Answer from the drawing. Dimensions are ordinates in mm from the lowest x, y and z of the part. A direction names the side the tool comes from. Give positions to 0.01 mm unless a question says otherwise; leave off trailing zeros. Order: outer loops, then holes, each group sorted by start corner. A loop starts at its lowest first (then second) coordinate and runs counter-clockwise, first axis right, second up. Notation, with made-up numbers: (64, 16) - (106, 16) arc R24 cw to (106, 32) - close; hole circle Ø9 at (74, 54.5). An arc over 180 degrees is marked (long way). Answer in a Markdown table with one row per item.
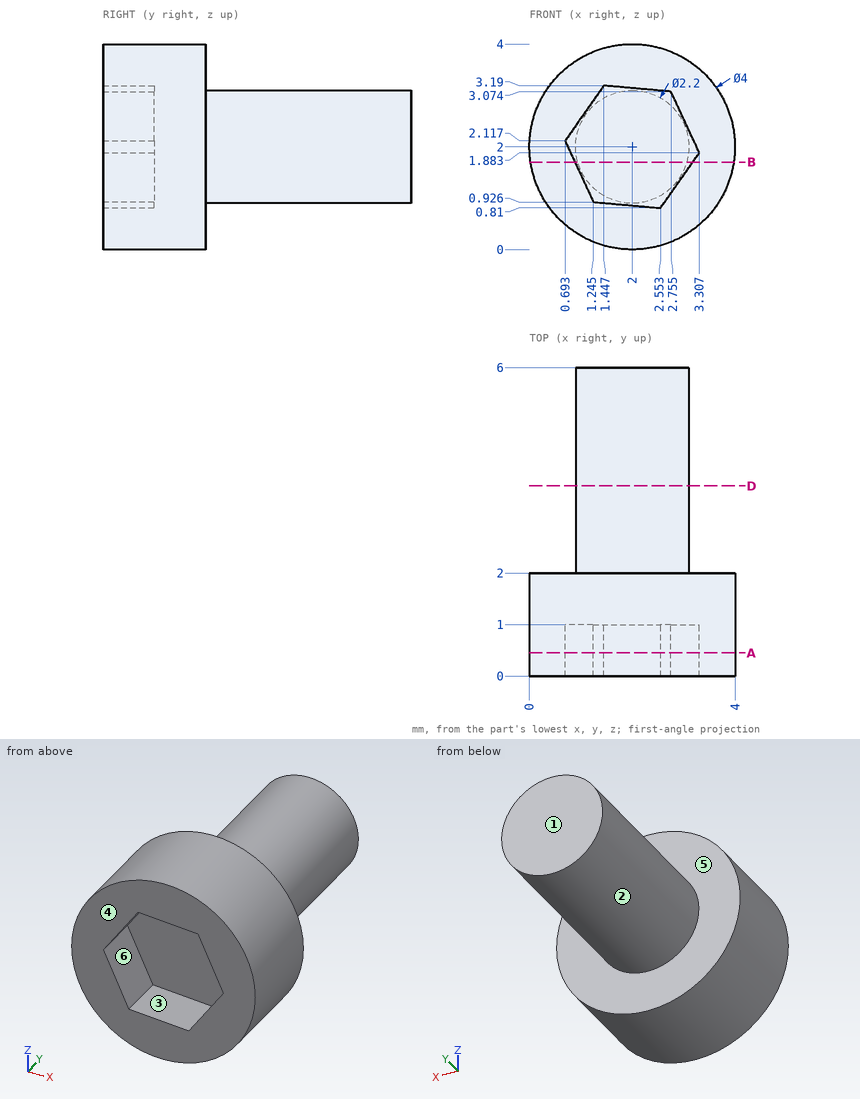
Item 1: Consider line 1 (Y direction, x = 1.2, z = 1.35); line 2 (Y direction, x = 3.4, z = 2.3); line 3 (Z direction, x = 1.2, y = 3.4) (1 decimal). Determine where each line is inside the solid, lowest interval first.
Answer block:
| item | result |
|---|---|
| line 1 | 1 to 6 |
| line 2 | 0 to 2 |
| line 3 | 1.2 to 2.8 |
Item 2: Find section B-B on z = 1.7. Write down the section's boundary in (x, y).
Answer block:
| item | result |
|---|---|
| outline | (0.02, 0) - (0.89, 0) - (0.89, 1) - (3.18, 1) - (3.18, 0) - (3.98, 0) - (3.98, 2) - (3.06, 2) - (3.06, 6) - (0.94, 6) - (0.94, 2) - (0.02, 2) - close |
Item 3: Find section A-A on y = 0.45. Write down the section's boundary in (x, z) (1 decimal).
Answer block:
| item | result |
|---|---|
| outline | circle Ø4 at (2, 2); hole (0.7, 2.1) - (1.2, 0.9) - (2.6, 0.8) - (3.3, 1.9) - (2.8, 3.1) - (1.4, 3.2) - close |
Item 4: Each of these flat-tipped pins is pushed along its axis until it touches: P1, Ø1.5, axis at x = 1, y = 5, coming from the -Z side; P2, Ø1.5, axis at y = 5, z = 1.5, coming from the -X side. Where does it stop, or does it pass through?
Answer block:
| item | result |
|---|---|
| P1 | z = 0.93 |
| P2 | x = 0.9 |
Item 5: Determine the mould class of the marked faces 1, 2 and 3 for opening direction X: pulls with the +X half, pulls with the -X half, needs draft (parallel to the pull), parting line crosses it, or undercut.
Answer block:
| item | result |
|---|---|
| face 1 | needs draft |
| face 2 | parting line crosses it |
| face 3 | undercut |
Item 6: Find section D-D on y = 3.7. Write down the section's boundary in (x, z).
Answer block:
| item | result |
|---|---|
| outline | circle Ø2.2 at (2, 2) |
Item 7: Which of the six approach directions +Z, -Z, +X, -X, +Y, -Y give full straight-line access (tool end or side, diameter ignored) to the marked faces 4, 5 and 6?
Answer block:
| item | result |
|---|---|
| face 4 | +Z, -Z, +X, -X, -Y |
| face 5 | +Y |
| face 6 | -Y |
